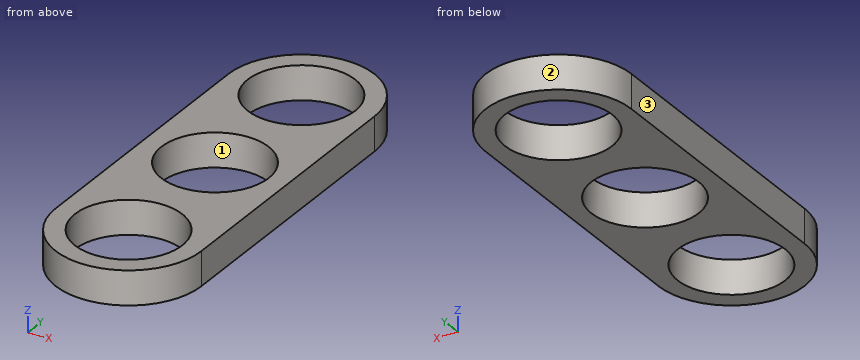
```python
from build123d import *

# Parameters (mm, degrees)
F0_R     = 11.05
F1_DEPTH = 7
F2_DEPTH = 7
F3_COUNT = 2


with BuildPart() as f1:
    # F0 (on Top) → F1 (new body)
    with BuildSketch(Plane.XY):
        with BuildLine():
            ThreePointArc((-15, 0), (0, -15), (15, 0))
            ThreePointArc((15, 0), (0, 15), (-15, 0))
        make_face()
        Circle(F0_R, mode=Mode.SUBTRACT)
    extrude(amount=F1_DEPTH)



with BuildPart() as f2:
    # F0 (on Top) → F2 (new body, through all)
    with BuildSketch(Plane.XY):
        with BuildLine():
            ThreePointArc((-15, 0), (0, 15), (15, 0))
            Line((15, 0), (15, 29.05))
            ThreePointArc((15, 29.05), (0, 44.05), (-15, 29.05))
            Line((-15, 29.05), (-15, 0))
        make_face()
        with Locations((0, 29.05)):
            Circle(F0_R, mode=Mode.SUBTRACT)
    extrude(amount=F2_DEPTH)


with BuildPart() as f1_1:
    add(f1.part)

    add(f2.part)  # F3 merges F2
    # F3: F2 ×2 about axis
    f3_axis = Axis((0, 0, 0), (0, 0, 1))
    for i in range(1, F3_COUNT):
        add(f2.part.rotate(f3_axis, i * 360 / F3_COUNT))


solid = f1_1.part
```
The listing builds one solid part. Answer for the finished solid, in the listing's coordinates (mm). Face numbers are marked on the shaded views. Round coordinates to 2 decimals unless told otherwise and drop trailing zeros. Loops run counter-clockwise (first coordinate to the right, second up) from the corner with the lowest first, then second, coordinate; pieces in that order, holes last.
Q1. Find the intervals of material crossed by line 1 (Y direction, x = 0, z = 4.5); line 2 (Y direction, x = -10, z = 2.5); line 3 (X direction, y = -31, z = 5.75), in increasing order.
Q2. For a pull along X with two mould halves and no side action, classify the marked faces 1, 2 and 3 as released by +X, released by -X, zero draft, split by the parting line, or undercut.
Q3. Given pin 1 Ø1.5 at (x, z) = (5, 2) entering from -Y; pin 2 Ø2 at (x, z) = (-3, 2) entering from +Y, each flat-ended and moving along its own axis, determine where each tip first touches the part or whether it passes through.
Q4. Section A-A, the plane y = 0 is taken. Determine the outline of the cut face in (x, z), then the cut area to 3 significant figures.
Q5. Section B-B, the plane x = 0 is taken. Determine the outline of the cut face in (y, z).
Q6. Section D-D, the plane y = -37.5 is taken. Determine the outline of the cut face in (x, z), then the cut area to 3 significant figures.
Q7. Section C-C, the plane z = 5.5 is taken. Determine the outline of the cut face in (x, y), then the cut area to 3 significant figures.
Completed:
1. line 1: y = -44.05 to -40.1, -18 to -11.05, 11.05 to 18, 40.1 to 44.05
1. line 2: y = -40.23 to -33.75, -24.35 to -4.7, 4.7 to 24.35, 33.75 to 40.23
1. line 3: x = -14.87 to -10.88, 10.88 to 14.87
2. face 1: undercut
2. face 2: split by the parting line
2. face 3: released by -X
3. pin 1: stops at y = -43.44
3. pin 2: stops at y = 43.92
4. outline: (-15, 0) - (-11.05, 0) - (-11.05, 7) - (-15, 7) - close; (11.05, 0) - (15, 0) - (15, 7) - (11.05, 7) - close
4. area: 55.3 mm2
5. outline: (-44.05, 0) - (-40.1, 0) - (-40.1, 7) - (-44.05, 7) - close; (-18, 0) - (-11.05, 0) - (-11.05, 7) - (-18, 7) - close; (11.05, 0) - (18, 0) - (18, 7) - (11.05, 7) - close; (40.1, 0) - (44.05, 0) - (44.05, 7) - (40.1, 7) - close
6. outline: (-12.39, 0) - (-7.12, 0) - (-7.12, 7) - (-12.39, 7) - close; (7.12, 0) - (12.39, 0) - (12.39, 7) - (7.12, 7) - close
6. area: 73.8 mm2
7. outline: (-15, -29.05) arc R15 ccw to (15, -29.05) - (15, 29.05) arc R15 ccw to (-15, 29.05) - close; hole circle Ø22.1 at (0, -29.05); hole circle Ø22.1 at (0, 0); hole circle Ø22.1 at (0, 29.05)
7. area: 1,300 mm2
